Design review of the part built by this model. Coordinates are the model's own, in mm. A direction names the side the tool comes from. Coordinates: 2 decimals unless noted, no trailing zeros. Order: outer loops, then holes, each group sorted by start corner. A loop starts at its lowest first (then second) coordinate and runs counter-clockwise, first axis right, second up. Notation, with made-up numbers: (68.5, 71) -> (87.5, 71) arc R21 ccw to (87.5, 91) -> close; hole circle Ø7 at (36.25, 81.5). An arc over 180 degrees is marked (long way). Write item = value, one per line.
```python
from build123d import *

# Parameters (mm, degrees)
SZKIC1_R                    = 3.000000079
DODANIE_WYCI_GNI_CIE1_DEPTH = 5
SZKIC2_W                    = 1.618528634
SZKIC2_H                    = 7.505645785
SZKIC2_W_2                  = 0.651830256
SZKIC2_H_2                  = 5.051684483
WYTNIJ_WYCI_GNI_CIE3_DEPTH  = 6


with BuildPart() as part:
    # Szkic1 → Dodanie-wyciągnięcie1 (new body)
    with BuildSketch(Plane.XY):
        with BuildLine():
            ThreePointArc((83.76241555, 5.522620658), (41.86347888, 6.752288216), (0, 4.635188213))
            ThreePointArc((0, 4.635188213), (-4.635188213, 0), (0, -4.635188213))
            ThreePointArc((0, -4.635188213), (41.86347888, -6.752288216), (83.76241555, -5.522620658))
            ThreePointArc((83.76241555, -5.522620658), (89.285036208, 0), (83.76241555, 5.522620658))
        make_face()
        with BuildLine():
            ThreePointArc((5.619311809, 4.445631254), (42.914384434, 5.983761034), (80.199446312, 4.219548453))
            ThreePointArc((80.199446312, 4.219548453), (78.239794892, 0), (80.199446312, -4.219548453))
            ThreePointArc((80.199446312, -4.219548453), (42.914384434, -5.983761034), (5.619311809, -4.445631254))
            ThreePointArc((5.619311809, -4.445631254), (4.261200111, -3.581390157), (4.194308577, -1.973004139))
            ThreePointArc((4.194308577, -1.973004139), (4.635188213, 0), (4.194308577, 1.973004139))
            ThreePointArc((4.194308577, 1.973004139), (4.261200111, 3.581390157), (5.619311809, 4.445631254))
        make_face(mode=Mode.SUBTRACT)
        with Locations((83.76241555, 0)):
            Circle(SZKIC1_R, mode=Mode.SUBTRACT)
        Circle(SZKIC1_R, mode=Mode.SUBTRACT)
    extrude(amount=DODANIE_WYCI_GNI_CIE1_DEPTH)

    # Szkic2 → Wytnij-wyciągnięcie3 (cut, through all)
    with BuildSketch(Plane.XY):
        with Locations((193.638606269, 0.381285041)):
            Rectangle(SZKIC2_W, SZKIC2_H)
        with Locations((-4.682734605, -0.038745932)):
            Rectangle(SZKIC2_W_2, SZKIC2_H_2)
    extrude(amount=WYTNIJ_WYCI_GNI_CIE3_DEPTH, mode=Mode.SUBTRACT)


solid = part.part
```
(1) The part is to be moulded in two halves that separate along Y. For faces 3 (the cylindrical face through (4.635, -0.029, 2.465)), 4 (the cylindrical face through (89.284, -0.121, 2.465)), 5 (the flat face through (-4.357, 0, 2)), say which applies: released by +Y, released by -Y, zero draft, split by the parting line, or undercut.
Report:
face_3 = undercut
face_4 = split by the parting line
face_5 = zero draft
(2) For L1, parallel to Y at x = 0, z = 3.95; L2, parallel to X at y = -0.5, z = 2.9; L3, parallel to X at y = -2.5, z = 1.55, list the stretches that pass through material, from the lowest coordinate up.
Report:
L1 = -4.64 to -3, 3 to 4.64
L2 = -4.36 to -2.96, 2.96 to 4.61, 78.26 to 80.8, 86.72 to 89.26
L3 = -3.9 to -1.66, 1.66 to 4.04, 78.84 to 82.1, 85.42 to 88.69
(3) We need section A-A (y = 0). Write out the cut boundary in (x, z).
Report:
outline = (-4.36, 0) -> (-3, 0) -> (-3, 5) -> (-4.36, 5) -> close; (3, 0) -> (4.64, 0) -> (4.64, 5) -> (3, 5) -> close; (78.24, 0) -> (80.76, 0) -> (80.76, 5) -> (78.24, 5) -> close; (86.76, 0) -> (89.29, 0) -> (89.29, 5) -> (86.76, 5) -> close
(4) We need section D-D (x = 55.5). Write out the cut boundary in (y, z), and give its area (3 significant figures).
Report:
outline = (-6.72, 0) -> (-5.76, 0) -> (-5.76, 5) -> (-6.72, 5) -> close; (5.76, 0) -> (6.72, 0) -> (6.72, 5) -> (5.76, 5) -> close
area = 9.62 mm²
(5) Insertion check: pin 1 (8 mm diameter, centred on x = 0, y = 0, fed in from -Z); pin 2 (5 mm diameter, centred on x = 27, y = 2.5, fed in from -Z); pin 3 (3 mm diameter, centred on y = 5, z = 4, fed in from -X). Each pin has a flat end and moves straight along its axis. Give the tip position at first contact, or say it passes through.
Report:
pin_1 = 0
pin_2 = through
pin_3 = -3.04
(6) For faces 1 (the flat face through (49.2, 6.6, 0)), 2 (the cylindrical face through (4.25, 3.56, 2.46)), list the 3-axis set-ups (+Z, -Z, +X, -X, +Y, -Y) from which the entire face can be reached by the end or side of a thin tool; tool diameter is ignored.
Report:
face_1 = -Z, +X, -X, +Y, -Y
face_2 = +Z, -Z
(7) We need section C-C (z = 2.45). Write out the cut boundary in (x, y).
Report:
outline = (-4.36, -1.58) arc R4.64 ccw to (0, -4.64) arc R524.96 ccw to (83.76, -5.52) arc R5.52 ccw to (83.76, 5.52) arc R524.96 ccw to (0, 4.64) arc R4.64 ccw to (-4.36, 1.58) -> close; hole circle Ø6 at (0, 0); hole (4.19, -1.97) arc R1.74 ccw to (5.62, -4.45) arc R421.91 ccw to (80.2, -4.22) arc R5.52 cw to (80.2, 4.22) arc R421.91 ccw to (5.62, 4.45) arc R1.74 ccw to (4.19, 1.97) arc R4.64 cw to start; hole circle Ø6 at (83.76, 0)
